```python
from build123d import *

# Parameters (mm, degrees)
SKETCH1_R           = 4
SKETCH1_R_2         = 2.5
BOSS_EXTRUDE1_DEPTH = 5
SKETCH2_R           = 0.75
CUT_EXTRUDE1_DEPTH  = 10


with BuildPart() as part:
    # Sketch1 → Boss-Extrude1 (new body)
    with BuildSketch(Plane.XY):
        with BuildLine():
            Line((-12.5, 6.822695454), (12.723447831, 4.317700065))
            ThreePointArc((12.723447831, 4.317700065), (17.5, -0.677304546), (12.723447831, -5.672309157))
            Line((12.723447831, -5.672309157), (-12.5, -8.177304546))
            ThreePointArc((-12.5, -8.177304546), (-20, -0.677304546), (-12.5, 6.822695454))
        make_face()
        with Locations((-12.5, -0.677304546)):
            Circle(SKETCH1_R, mode=Mode.SUBTRACT)
        with Locations((12.5, -0.677304546)):
            Circle(SKETCH1_R_2, mode=Mode.SUBTRACT)
    extrude(amount=BOSS_EXTRUDE1_DEPTH)

    # Sketch2 → Cut-Extrude1 (cut)
    with BuildSketch(Plane.XY.offset(5)):
        with Locations((-3.750139294, -0.627932239)):
            Circle(SKETCH2_R)
        with Locations((2.24976519, -0.594076942)):
            Circle(SKETCH2_R)
    extrude(amount=-CUT_EXTRUDE1_DEPTH, mode=Mode.SUBTRACT)


solid = part.part
```
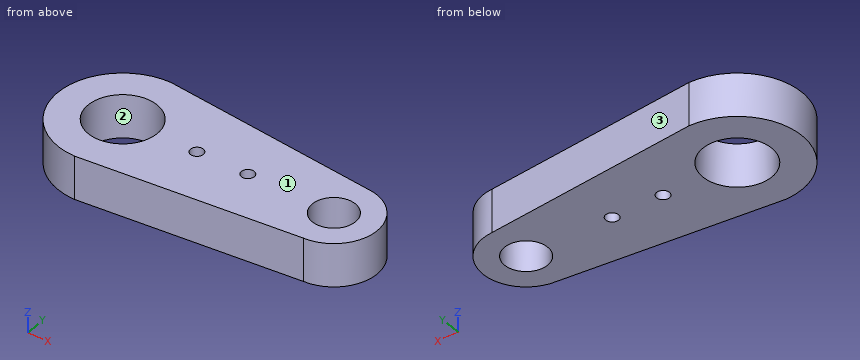
CAD build for the part. Positions are in the model's coordinates, mm. Face numbers are marked on the shaded views. Round coordinates to 2 decimals unless told otherwise and drop trailing zeros. Loops run counter-clockwise (first coordinate to the right, second up) from the corner with the lowest first, then second, coordinate; pieces in that order, holes last. Notation, with made-up numbers: M 75.25,77 L 84.25,77 A13 ccw 84.25,92 Z; hole C -37,-34.75 d9. An arc over 180 degrees is marked long. Return JSON: item names as keys, results as strings. Group by question number.
(1) Saw through at C-C, the plane z = 2.15. List the corners of the cut face in (x, y).
(2) Saw through at B-B, the plane y = 2.25. List the corners of the cut face in (x, z), and give its area (3 significant figures).
(3) Drop flat-ended pins along their axis: P1, Ø3, axis at y = 0, z = 1.5, coming from the +X side; P2, Ø1, axis at y = -5, z = 3, coming from the -X side; P3, Ø3, axis at y = 3.5, z = 3, coming from the -X side; P4, Ø1.4, axis at x = 2.25, y = -0.59, coming from the -Z side. Give the stop position or say it passes through.
(4) Saw through at A-A, the plane x = 14. List the corners of the cut face in (y, z), and give its area (3 significant figures).
(5) Mould opens along X. For the marked faces 1, 2 and 3 say: +X half, -X half, draft (parallel to the pull), parting line (faces both ways), or undercut.
(6) Wall check: probe 1 along Y at (x, z) = (-12.5, 1.9); probe 2 along X at (y, z) = (1, 4.75); probe 3 along Y at (x, z) = (15.5, 3.7). Give the ranges that are in metal, low to high. Write a range as [from, to].
(7) Saw through at D-D, the plane y = -6.5. List the corners of the cut face in (x, z).
Answer list:
{
 "1": {"outline": "M -12.5,-8.18 L 12.72,-5.67 A5 ccw 12.72,4.32 L -12.5,6.82 A7.5 ccw Z; hole C -12.5,-0.68 d8; hole C -3.75,-0.63 d1.5; hole C 2.25,-0.59 d1.5; hole C 12.5,-0.68 d5"},
 "2": {"outline": "M -19.41,0 L -15.23,0 L -15.23,5 L -19.41,5 Z; M -9.77,0 L 16.55,0 L 16.55,5 L -9.77,5 Z", "area": "153 mm2"},
 "3": {"P1": "x = 17.5", "P2": "x = -18.95", "P3": "x = -19.51", "P4": "through"},
 "4": {"outline": "M -5.45,0 L -2.68,0 L -2.68,5 L -5.45,5 Z; M 1.32,0 L 4.09,0 L 4.09,5 L 1.32,5 Z", "area": "27.7 mm2"},
 "5": {"face 1": "draft", "face 2": "undercut", "face 3": "+X half"},
 "6": {"probe 1": "[-8.18, -4.68], [3.32, 6.82]", "probe 2": "[-19.81, -16.13], [-8.87, 10.65], [14.35, 17.21]", "probe 3": "[-4.68, 3.32]"},
 "7": {"outline": "M -17.23,0 L 4.39,0 L 4.39,5 L -17.23,5 Z"}
}
